Can you work these out from the model? Positions are in its coordinate system, mm. Face numbers are marked on the shaded views. A direction names the side the tool comes from. Round coordinates to 2 decimals unless told otherwise and drop trailing zeros. Write each loop counter-clockwise with the first axis right and the second up, starting at its lowest first coordinate (ties: lowest second). Pieces come first, ordered by that corner, then holes.
Q1. I'm going to push flat-ended pins straight in: pin 1 Ø10 at (x, z) = (-32.5, -19) entering from +Y; pin 2 Ø0.8 at (x, y) = (-17, 0.5) entering from +Z. Where does each tip first touch, or does it pass through?
Q2. Please list where these lines run through material, in increasing order: line 1 along X through (y, z) = (-1.65, 32.8); line 2 along Z through (x, y) = (19.5, -3.5); line 3 along Z through (x, y) = (5, -2.1).
Q3. If we section it at A-A (z = 12.2): Please give me the cut outline in (x, y).
Q4. If we section it at D-D (z = -8): Please give me the cut outline in (x, y).
Q5. If we section it at B-B (x = 7): Please give me the cut outline in (y, z), plus the area to 3 significant figures.
Q6. For the marked faces 1 and 2, which set-ups out of +Z, -Z, +X, -X, +Y, -Y let a thin tool reach every point of the face, with its end or its side?
Q7. If we section it at C-C (y = -2.15): Give the number of separate pieces and of enclosed holes in the cut face, plus the area to 3 significant figures.
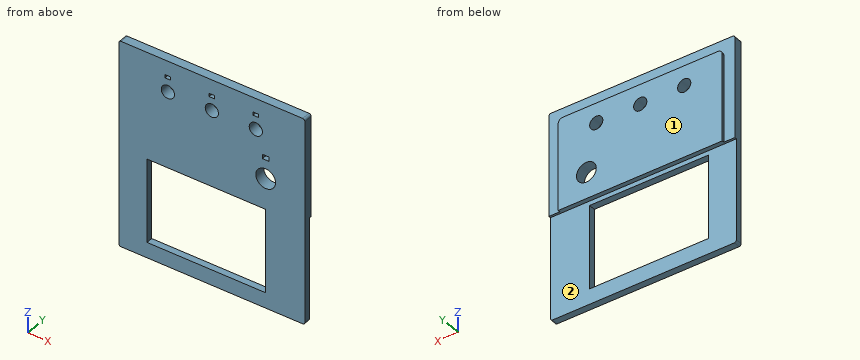
from build123d import *

# Parameters (mm, degrees)
SKETCH_1_W          = 74.6
SKETCH_1_H          = 83.6
EXTRUDE_1_DEPTH     = 1
FILLET_1_R          = 2
SKETCH_2_W          = 84.6
SKETCH_2_H          = 93.6
EXTRUDE_2_DEPTH     = 4
FILLET_2_R          = 1
SKETCH_3_R          = 3
SKETCH_3_R_2        = 4.5
SKETCH_3_W          = 54
SKETCH_3_H          = 38
CUT_EXTRUDE_1_DEPTH = 64.281355864
SKETCH_4_W          = 84.6
SKETCH_4_H          = 47
CUT_EXTRUDE_2_DEPTH = 2
SKETCH_5_W          = 2.5
SKETCH_5_H          = 1.5
SKETCH_5_W_2        = 3
SKETCH_5_H_2        = 2
CUT_EXTRUDE_3_DEPTH = 3.6


with BuildPart() as part:
    # Эскиз1 → Бобышка-Вытянуть1 (new body)
    with BuildSketch(Plane(origin=(0, 0, 0), x_dir=(1, 0, 0), z_dir=(0, 1, 0))):
        Rectangle(SKETCH_1_W, SKETCH_1_H)
    extrude(amount=EXTRUDE_1_DEPTH)

    # Скругление1
    fillet_1_edges = [part.edges().sort_by_distance(p)[0] for p in [
        (37.3, 0.5, 41.8),
        (-37.3, 0.5, 41.8),
        (-37.3, 0.5, -41.8),
        (37.3, 0.5, -41.8),
    ]]
    fillet(fillet_1_edges, radius=FILLET_1_R)

    # Эскиз2 → Бобышка-Вытянуть2 (add)
    with BuildSketch(Plane.XZ):
        Rectangle(SKETCH_2_W, SKETCH_2_H)
    extrude(amount=EXTRUDE_2_DEPTH)

    # Скругление2
    fillet_2_edges = [part.edges().sort_by_distance(p)[0] for p in [
        (-42.3, -2, 46.8),
        (-42.3, -2, -46.8),
        (42.3, -2, -46.8),
        (42.3, -2, 46.8),
    ]]
    fillet(fillet_2_edges, radius=FILLET_2_R)

    # Эскиз3 → Вырез-Вытянуть1 (cut, through all)
    with BuildSketch(Plane(origin=(0, 1, 0), x_dir=(1, 0, 0), z_dir=(0, 1, 0))):
        with Locations(Location((-20, -32.8, 0), (0, 0, 270))):
            Circle(SKETCH_3_R)
        with Locations(Location((0, -32.8, 0), (0, 0, 270))):
            Circle(SKETCH_3_R)
        with Locations(Location((20, -32.8, 0), (0, 0, 270))):
            Circle(SKETCH_3_R)
        with Locations(Location((24.5, -12.2, 0), (0, 0, 270))):
            Circle(SKETCH_3_R_2)
        with Locations((-2.5, 20.8)):
            Rectangle(SKETCH_3_W, SKETCH_3_H)
    extrude(amount=-CUT_EXTRUDE_1_DEPTH, mode=Mode.SUBTRACT)

    # Эскиз4 → Вырез-Вытянуть2 (cut)
    with BuildSketch(Plane(origin=(0, 1, 0), x_dir=(1, 0, 0), z_dir=(0, 1, 0))):
        with Locations((0, 23.3)):
            Rectangle(SKETCH_4_W, SKETCH_4_H)
    extrude(amount=-CUT_EXTRUDE_2_DEPTH, mode=Mode.SUBTRACT)

    # Эскиз5 → Вырез-Вытянуть3 (cut)
    with BuildSketch(Plane.XZ.offset(4)):
        with Locations((-20, 39.418347297)):
            Rectangle(SKETCH_5_W, SKETCH_5_H)
        with Locations((0, 39.418347297)):
            Rectangle(SKETCH_5_W, SKETCH_5_H)
        with Locations((20, 39.418347297)):
            Rectangle(SKETCH_5_W, SKETCH_5_H)
        with Locations((24.5, 21.7)):
            Rectangle(SKETCH_5_W_2, SKETCH_5_H_2)
    extrude(amount=-CUT_EXTRUDE_3_DEPTH, mode=Mode.SUBTRACT)


solid = part.part
A:
1. pin 1: stops at y = -1
1. pin 2: stops at z = 41.8
2. line 1: x = -42.3 to -23, -17 to -3, 3 to 17, 23 to 42.3
2. line 2: z = -46.8 to -39.8, -1.8 to 29.84, 35.76 to 38.67, 40.17 to 46.8
2. line 3: z = -46.8 to -39.8, -1.8 to 46.8
3. outline: (-42.3, -4) - (20, -4) - (20, 1) - (-37.3, 1) - (-37.3, 0) - (-42.3, 0) - close; (29, -4) - (42.3, -4) - (42.3, 0) - (37.3, 0) - (37.3, 1) - (29, 1) - close
4. outline: (-42.3, -4) - (-29.5, -4) - (-29.5, -1) - (-42.3, -1) - close; (24.5, -4) - (42.3, -4) - (42.3, -1) - (24.5, -1) - close
5. outline: (-4, -46.8) - (-1, -46.8) - (-1, -39.8) - (-4, -39.8) - close; (-4, -1.8) - (-1, -1.8) - (-1, 0.2) - (1, 0.2) - (1, 41.8) - (0, 41.8) - (0, 46.8) - (-4, 46.8) - close
5. area: 255 mm2
6. face 1: +Z, -Z, +X, -X, +Y
6. face 2: -Z, +X, -X, +Y
7. separate pieces: 1
7. enclosed holes: 9
7. area: 5,700 mm2
